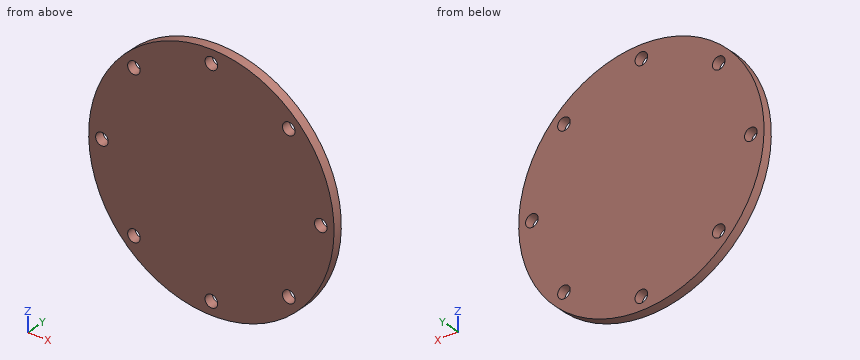
```python
from build123d import *

# Parameters (mm, degrees)
SKETCH_1_R          = 195
EXTRUDE_1_DEPTH     = 15
CUT_EXTRUDE_1_REACH = 278.179
SKETCH_2_R          = 10


with BuildPart() as part:
    # 草图1 → 凸台-拉伸1 (new body)
    with BuildSketch(Plane(origin=(0, 0, 0), x_dir=(1, 0, 0), z_dir=(0, 1, 0))):
        with Locations(Location((0, 0, 0), (0, 0, 270))):
            Circle(SKETCH_1_R)
    extrude(amount=EXTRUDE_1_DEPTH)

    # 草图2 → 切除-拉伸1 (cut, up to next)
    with BuildSketch(Plane(origin=(0, 15, 0), x_dir=(1, 0, 0), z_dir=(0, 1, 0)), mode=Mode.PRIVATE) as cut_extrude_1_sk1:
        with Locations(Location((-174, 0, 0), (0, 0, 270))):
            Circle(SKETCH_2_R)
    cut_extrude_1_tool1 = extrude(cut_extrude_1_sk1.sketch, amount=-CUT_EXTRUDE_1_REACH, mode=Mode.PRIVATE) & part.part
    # 草图2 → 切除-拉伸1 (cut, up to next)
    with BuildSketch(Plane(origin=(0, 15, 0), x_dir=(1, 0, 0), z_dir=(0, 1, 0)), mode=Mode.PRIVATE) as cut_extrude_1_sk2:
        with Locations(Location((-123.036579926, 123.036579926, 0), (0, 0, 270))):
            Circle(SKETCH_2_R)
    cut_extrude_1_tool2 = extrude(cut_extrude_1_sk2.sketch, amount=-CUT_EXTRUDE_1_REACH, mode=Mode.PRIVATE) & part.part
    # 草图2 → 切除-拉伸1 (cut, up to next)
    with BuildSketch(Plane(origin=(0, 15, 0), x_dir=(1, 0, 0), z_dir=(0, 1, 0)), mode=Mode.PRIVATE) as cut_extrude_1_sk3:
        with Locations(Location((0, 174, 0), (0, 0, 270))):
            Circle(SKETCH_2_R)
    cut_extrude_1_tool3 = extrude(cut_extrude_1_sk3.sketch, amount=-CUT_EXTRUDE_1_REACH, mode=Mode.PRIVATE) & part.part
    # 草图2 → 切除-拉伸1 (cut, up to next)
    with BuildSketch(Plane(origin=(0, 15, 0), x_dir=(1, 0, 0), z_dir=(0, 1, 0)), mode=Mode.PRIVATE) as cut_extrude_1_sk4:
        with Locations(Location((123.036579926, 123.036579926, 0), (0, 0, 270))):
            Circle(SKETCH_2_R)
    cut_extrude_1_tool4 = extrude(cut_extrude_1_sk4.sketch, amount=-CUT_EXTRUDE_1_REACH, mode=Mode.PRIVATE) & part.part
    # 草图2 → 切除-拉伸1 (cut, up to next)
    with BuildSketch(Plane(origin=(0, 15, 0), x_dir=(1, 0, 0), z_dir=(0, 1, 0)), mode=Mode.PRIVATE) as cut_extrude_1_sk5:
        with Locations(Location((174, 0, 0), (0, 0, 270))):
            Circle(SKETCH_2_R)
    cut_extrude_1_tool5 = extrude(cut_extrude_1_sk5.sketch, amount=-CUT_EXTRUDE_1_REACH, mode=Mode.PRIVATE) & part.part
    # 草图2 → 切除-拉伸1 (cut, up to next)
    with BuildSketch(Plane(origin=(0, 15, 0), x_dir=(1, 0, 0), z_dir=(0, 1, 0)), mode=Mode.PRIVATE) as cut_extrude_1_sk6:
        with Locations(Location((123.036579926, -123.036579926, 0), (0, 0, 270))):
            Circle(SKETCH_2_R)
    cut_extrude_1_tool6 = extrude(cut_extrude_1_sk6.sketch, amount=-CUT_EXTRUDE_1_REACH, mode=Mode.PRIVATE) & part.part
    # 草图2 → 切除-拉伸1 (cut, up to next)
    with BuildSketch(Plane(origin=(0, 15, 0), x_dir=(1, 0, 0), z_dir=(0, 1, 0)), mode=Mode.PRIVATE) as cut_extrude_1_sk7:
        with Locations(Location((0, -174, 0), (0, 0, 270))):
            Circle(SKETCH_2_R)
    cut_extrude_1_tool7 = extrude(cut_extrude_1_sk7.sketch, amount=-CUT_EXTRUDE_1_REACH, mode=Mode.PRIVATE) & part.part
    # 草图2 → 切除-拉伸1 (cut, up to next)
    with BuildSketch(Plane(origin=(0, 15, 0), x_dir=(1, 0, 0), z_dir=(0, 1, 0)), mode=Mode.PRIVATE) as cut_extrude_1_sk8:
        with Locations(Location((-123.036579926, -123.036579926, 0), (0, 0, 270))):
            Circle(SKETCH_2_R)
    cut_extrude_1_tool8 = extrude(cut_extrude_1_sk8.sketch, amount=-CUT_EXTRUDE_1_REACH, mode=Mode.PRIVATE) & part.part
    add(cut_extrude_1_tool1.solids().sort_by_distance((-174, 15, 0))[0], mode=Mode.SUBTRACT)
    add(cut_extrude_1_tool2.solids().sort_by_distance((-123.03658, 15, -123.03658))[0], mode=Mode.SUBTRACT)
    add(cut_extrude_1_tool3.solids().sort_by_distance((0, 15, -174))[0], mode=Mode.SUBTRACT)
    add(cut_extrude_1_tool4.solids().sort_by_distance((123.03658, 15, -123.03658))[0], mode=Mode.SUBTRACT)
    add(cut_extrude_1_tool5.solids().sort_by_distance((174, 15, 0))[0], mode=Mode.SUBTRACT)
    add(cut_extrude_1_tool6.solids().sort_by_distance((123.03658, 15, 123.03658))[0], mode=Mode.SUBTRACT)
    add(cut_extrude_1_tool7.solids().sort_by_distance((0, 15, 174))[0], mode=Mode.SUBTRACT)
    add(cut_extrude_1_tool8.solids().sort_by_distance((-123.03658, 15, 123.03658))[0], mode=Mode.SUBTRACT)


solid = part.part
```
Design review of the part built by this model. Coordinates are the model's own, in mm. Coordinates: 2 decimals unless noted, no trailing zeros. Order: outer loops, then holes, each group sorted by start corner. A loop starts at its lowest first (then second) coordinate and runs counter-clockwise, first axis right, second up. Notation, with made-up numbers: (-22, 39.5) - (3, 39.5) arc R33 cw to (3, 67.5) - close; hole circle Ø11 at (66, 35.25). An arc over 180 degrees is marked (long way). One line per question, with ' | ' between items.
Q1. Consider section B-B, the plane x = 0. Give the boundary of the cut face in (y, z).
Answer key:
outline: (0, -195) - (15, -195) - (15, -184) - (0, -184) - close; (0, -164) - (15, -164) - (15, 164) - (0, 164) - close; (0, 184) - (15, 184) - (15, 195) - (0, 195) - close
Q2. Consider section A-A, the plane z = 0. Give the boundary of the cut face in (x, y).
Answer key:
outline: (-195, 0) - (-184, 0) - (-184, 15) - (-195, 15) - close; (-164, 0) - (164, 0) - (164, 15) - (-164, 15) - close; (184, 0) - (195, 0) - (195, 15) - (184, 15) - close
Q3. To check wall thickness, follow line 1 along X through (y, z) = (4.25, 0); line 2 along Z through (x, y) = (-131, 4.5); line 3 along X through (y, z) = (13.5, 123). State the ranges of each line that lie inside material, in increasing order.
Answer key:
line 1: x = -195 to -184, -164 to 164, 184 to 195 | line 2: z = -144.44 to -129.09, -116.99 to 116.99, 129.09 to 144.44 | line 3: x = -151.31 to -133.04, -113.04 to 113.04, 133.04 to 151.31
Q4. Clearance check with flat-ended pins moving along their axes: pin 1 Ø1 at (y, z) = (12, 114) entering from +X; pin 2 Ø5 at (x, y) = (99, 3) entering from +Z; pin 3 Ø5 at (y, z) = (2, -24.5) entering from -X (3 decimals). State where each tip first meets the part, or that it passes through.
Answer key:
pin 1: stops at x = 158.56 | pin 2: stops at z = 169.45 | pin 3: stops at x = -193.755
Q5. Consider section C-C, the plane y = 8.5. Give the number of separate pieces and of enclosed holes in the cut face, then the cut area to 3 significant figures.
Answer key:
separate pieces: 1 | enclosed holes: 8 | area: 117,000 mm2
Q6. Consider section D-D, the plane x = 174. Give the boundary of the cut face in (y, z).
Answer key:
outline: (0, -88.03) - (15, -88.03) - (15, -10) - (0, -10) - close; (0, 10) - (15, 10) - (15, 88.03) - (0, 88.03) - close
